For this review, take the finished solid that the model builds, in its own axes (mm). A direction names the side the tool comes from. Give positions to 0.01 mm unless a question says otherwise; leave off trailing zeros. Loops run counter-clockwise (first coordinate to the right, second up) from the corner with the lowest first, then second, coordinate; pieces in that order, holes last.
```python
from build123d import *

# Parameters (mm, degrees)
F4_DEPTH       = 5
F5_DEPTH       = 20
F7_D           = 3.3
F7_CBORE_D     = 6.5
F7_CBORE_DEPTH = 3


# Not quite as in the source:
# - the program builds the solid bodies; features that only make, move or delete a surface that nothing else refers to are left out


with BuildPart() as f4:
    # F3 (on Top) → F4 (new body)
    with BuildSketch(Plane.XY):
        Polygon((-193.5, 232.5), (-193.5, 237.5), (-243.5, 237.5), (-243.5, 187.5), (-238.5, 187.5), (-238.5, 204), (-238.5, 232.5), (-210, 232.5), align=None)
        with BuildLine():
            Line((-210, 214), (-210, 232.5))
            Line((-210, 232.5), (-238.5, 232.5))
            Line((-238.5, 232.5), (-238.5, 204))
            Line((-238.5, 204), (-220, 204))
            ThreePointArc((-220, 204), (-227.0710678119, 221.0710678119), (-210, 214))
        make_face()
        with BuildLine():
            ThreePointArc((-220, 204), (-212.9289321881, 206.9289321881), (-210, 214))
            ThreePointArc((-210, 214), (-227.0710678119, 221.0710678119), (-220, 204))
        make_face()
    extrude(amount=F4_DEPTH)

    # F3 (on Top) → F5 (join)
    with BuildSketch(Plane.XY):
        Polygon((-193.5, 232.5), (-193.5, 237.5), (-243.5, 237.5), (-243.5, 187.5), (-238.5, 187.5), (-238.5, 204), (-238.5, 232.5), (-210, 232.5), align=None)
    extrude(amount=F5_DEPTH)

    # F7 (through all)
    with Locations(Plane.XY.offset(5)):
        with Locations((-232, 226), (-220, 214)):
            CounterBoreHole(F7_D / 2, F7_CBORE_D / 2, F7_CBORE_DEPTH)


solid = f4.part
```
Item 1: Take a section at B-B on z = 3.25. Give the boundary of the cut face in (x, y), and give its area (3 significant figures).
Answer:
outline: (-243.5, 187.5) - (-238.5, 187.5) - (-238.5, 204) - (-220, 204) arc R10 ccw to (-210, 214) - (-210, 232.5) - (-193.5, 232.5) - (-193.5, 237.5) - (-243.5, 237.5) - close; hole circle Ø6.5 at (-232, 226); hole circle Ø6.5 at (-220, 214)
area: 1,200 mm2
Item 2: For L1, parallel to X at y = 214, z = 1.1; L2, parallel to X at y = 214, z = 3.65; L3, parallel to Y at x = -232, z = 1.1, list the stretches that pass through material, from the lowest coordinate up.
Answer:
L1: x = -243.5 to -221.65, -218.35 to -210
L2: x = -243.5 to -223.25, -216.75 to -210
L3: y = 204 to 224.35, 227.65 to 237.5
Item 3: Clearance check with flat-ended pins moving along their axes: pin 1 Ø4 at (x, y) = (-206.5, 221.5) entering from +Z; pin 2 Ø10.5 at (x, y) = (-232, 226) entering from +Z; pin 3 Ø12 at (y, z) = (208, 8) entering from +X; pin 4 Ø3 at (x, y) = (-220, 214.5) entering from +Z. State where each tip first meets the part, or that it passes through.
Answer:
pin 1: passes through
pin 2: stops at z = 5
pin 3: stops at x = -210.03
pin 4: stops at z = 2
Item 4: Take a section at A-A on x = -232. Give the boundary of the cut face in (y, z), and give its area (3 significant figures).
Answer:
outline: (204, 0) - (224.35, 0) - (224.35, 2) - (222.75, 2) - (222.75, 5) - (204, 5) - close; (227.65, 0) - (237.5, 0) - (237.5, 20) - (232.5, 20) - (232.5, 5) - (229.25, 5) - (229.25, 2) - (227.65, 2) - close
area: 216 mm2
Item 5: The part is to be moulded in two halves that separate along X. For faces 6 (the cylindrical face through (-232.423, 229.222, 3.521)), 7 (the flat face through (-239, 224, 20)), 8 (the flat face through (-238.5, 210, 12)), say which applies: released by +X, released by -X, zero draft, split by the parting line, or undercut.
Answer:
face 6: undercut
face 7: zero draft
face 8: released by +X
Item 6: Take a section at C-C on y = 227. Give the boundary of the cut face in (x, z), and give its area (3 significant figures).
Answer:
outline: (-243.5, 0) - (-233.31, 0) - (-233.31, 2) - (-235.09, 2) - (-235.09, 5) - (-238.5, 5) - (-238.5, 20) - (-243.5, 20) - close; (-230.69, 0) - (-210, 0) - (-210, 5) - (-228.91, 5) - (-228.91, 2) - (-230.69, 2) - close
area: 219 mm2
Item 7: Tool access review of faces 1 (the flat face through (-224, 218, 5)), 2 (the flat face through (-218.6, 212.6, 2)), 3 (the flat face through (-224, 218, 0)), 4 (the flat face through (-210, 223, 2)), 5 (the flat face through (-193.5, 235, 10)): name each direction out of +Z, -Z, +X, -X, +Y, -Y from which nothing blocks a thin tool from reaching the whole face with its end or side.
Answer:
face 1: +Z, +X, -Y
face 2: +Z
face 3: -Z, +X, -X, +Y, -Y
face 4: +Z, -Z, +X, -Y
face 5: +Z, -Z, +X, +Y, -Y
Item 8: Take a section at D-D on z = 7.75. Give the boundary of the cut face in (x, y).
Answer:
outline: (-243.5, 187.5) - (-238.5, 187.5) - (-238.5, 232.5) - (-193.5, 232.5) - (-193.5, 237.5) - (-243.5, 237.5) - close
